```python
from build123d import *

# Parameters (mm, degrees)
F0_W          = 25.4
F0_H          = 25.4
F1_DEPTH      = 5.08
F3_DEPTH      = 25.4
F5_DEPTH      = 25.4
F6_R          = 1.27
F7_DEPTH      = 25.4
F7_DEPTH_BACK = 25.4
F9_DEPTH      = 3.81
F10_R         = 1.27
F11_DEPTH     = 3.175


with BuildPart() as f1:
    # F0 (on Top) → F1 (new body)
    with BuildSketch(Plane.XY):
        Rectangle(F0_W, F0_H)
    extrude(amount=F1_DEPTH)

    # F2 (on face) → F3 (join)
    with BuildSketch(Plane(origin=(-12.7, 0, 0), x_dir=(0, -1, 0), z_dir=(-1, 0, 0))):
        with BuildLine():
            Line((-1.143, 5.08), (1.143, 5.08))
            ThreePointArc((1.143, 5.08), (0, 6.223), (-1.143, 5.08))
        make_face()
    extrude(amount=-F3_DEPTH)

    # F4 (on face) → F5 (join)
    with BuildSketch(Plane.XZ.offset(12.7)):
        with BuildLine():
            Line((-1.143, 5.08), (1.143, 5.08))
            ThreePointArc((1.143, 5.08), (0, 6.223), (-1.143, 5.08))
        make_face()
    extrude(amount=-F5_DEPTH)

    # F6 (on face) → F7 (cut, two sides)
    with BuildSketch(Plane.XY.offset(5.08)) as f7_sk:
        Circle(F6_R)
    extrude(amount=-F7_DEPTH, mode=Mode.SUBTRACT)
    extrude(f7_sk.sketch, amount=F7_DEPTH_BACK, mode=Mode.SUBTRACT)

    # F8 (on face) → F9 (join)
    with BuildSketch(Plane.XY.offset(5.08)):
        Polygon((12.7, -1.143), (6.9215, -6.9215), (12.7, -12.7), align=None)
    extrude(amount=F9_DEPTH)

    # F10 (on face) → F11 (cut)
    with BuildSketch(Plane(origin=(0, 0, 0), x_dir=(1, 0, 0), z_dir=(0, 0, -1))):
        Polygon((-1.8330871047, -3.175), (1.8330871047, -3.175), (3.6661742094, 0), (1.8330871047, 3.175), (-1.8330871047, 3.175), (-3.6661742094, 0), align=None)
        Circle(F10_R, mode=Mode.SUBTRACT)
    extrude(amount=-F11_DEPTH, mode=Mode.SUBTRACT)


solid = f1.part
```
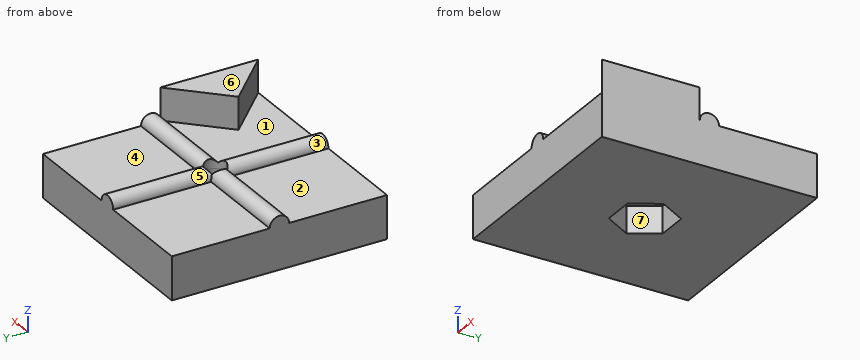
CAD build for the part. Positions are in the model's coordinates, mm. Face numbers are marked on the shaded views. A direction names the side the tool comes from. Round coordinates to 2 decimals unless told otherwise and drop trailing zeros. Loops run counter-clockwise (first coordinate to the right, second up) from the corner with the lowest first, then second, coordinate; pieces in that order, holes last. Notation, with made-up numbers: M 18.5,71.25 L 66.5,71.25 A25 ccw 66.5,103.25 Z; hole C -30,2.25 d1. An arc over 180 degrees is marked long. Return JSON: item names as keys, results as strings. Group by question number.
(1) Saw through at B-B, the plane z = 1. List the corners of the cut face in (x, y) (3 decimals).
(2) Saw through at C-C, the plane y = -5. List the corners of the cut face in (x, z), and give its area (3 significant figures).
(3) Wall check: probe 1 along X at (y, z) = (0, 3.6); probe 2 along Z at (x, y) = (6.75, 8). Give the ranges that are in metal, low to high. Write a range as [from, to].
(4) Mould opens along X. For the marked faces 5, 6 and 7 say: +X half, -X half, draft (parallel to the pull), parting line (faces both ways), or undercut.
(5) Saw through at D-D, the plane x = 9. List the corners of the cut face in (y, z).
(6) Drop flat-ended pins along their axis: P1, Ø2, axis at x = 0, y = 0, coming from the -Z side; P2, Ø8, axis at x = -10, y = -4, coming from the +Z side; P3, Ø1, axis at y = 1.5, z = 5.5, coming from the -X side; P4, Ø9, axis at x = 5, y = 9, coming from the +Z side. Give the stop position or say it passes through.
(7) Saw through at A-A, the plane x = 0. List the corners of the cut face in (y, z) (3 decimals).
(8) Tool access for the marked faces 1, 2, 3 and 4: list every direction of +Z, -Z, +X, -X, +Y, -Y with a clear straight run to the whole face (end or side of a thin tool).
Answer list:
{
 "1": {"outline": "M -12.7,-12.7 L 12.7,-12.7 L 12.7,12.7 L -12.7,12.7 Z; hole M -3.666,0 L -1.833,-3.175 L 1.833,-3.175 L 3.666,0 L 1.833,3.175 L -1.833,3.175 Z"},
 "2": {"outline": "M -12.7,0 L 12.7,0 L 12.7,8.89 L 8.84,8.89 L 8.84,5.08 L 1.14,5.08 A1.14 ccw -1.14,5.08 L -12.7,5.08 Z", "area": "146 mm2"},
 "3": {"probe 1": "[-12.7, -1.27], [1.27, 12.7]", "probe 2": "[0, 5.08]"},
 "4": {"face 5": "parting line", "face 6": "draft", "face 7": "undercut"},
 "5": {"outline": "M -12.7,0 L 12.7,0 L 12.7,5.08 L 1.14,5.08 A1.14 ccw -1.14,5.08 L -4.84,5.08 L -4.84,8.89 L -9,8.89 L -9,5.08 L -12.7,5.08 Z"},
 "6": {"P1": "through", "P2": "z = 6.22", "P3": "x = -12.7", "P4": "z = 6.11"},
 "7": {"outline": "M -12.7,0 L -3.175,0 L -3.175,3.175 L -1.27,3.175 L -1.27,6.223 L -12.7,6.223 Z; M 1.27,3.175 L 3.175,3.175 L 3.175,0 L 12.7,0 L 12.7,6.223 L 1.27,6.223 Z"},
 "8": {"face 1": "+Z", "face 2": "+Z, -X, -Y", "face 3": "+Z, -Y", "face 4": "+Z, +X, +Y"}
}
